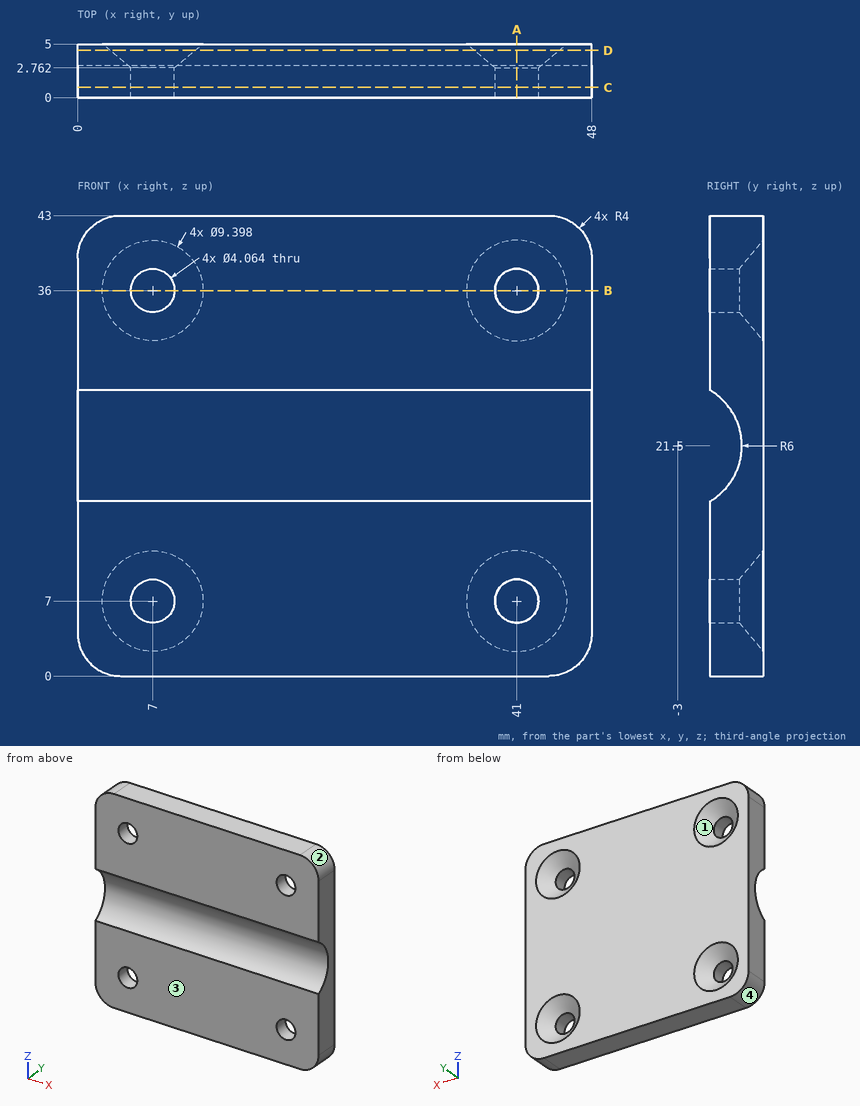
Verification items for this drawing (mm, ordinates from the low corner). Coordinates: 2 decimals unless noted, no trailing zeros. Loops run counter-clockwise (first coordinate to the right, second up) from the corner with the lowest first, then second, coordinate; pieces in that order, holes last.
Item 1: Sectioned sample at C-C, the plane y = 0.95. Record the boundary of the cut face in (x, z), then the cut area to 3 significant figures.
Item 2: Go/stop test with a flat-tipped pin: pin 1 Ø4.5 at (x, z) = (7, 7) entering from -Y. Record where the tip stops, or that it passes through.
Item 3: Release check for a two-part mould opening along Z. For the marked faces 1, 2, 3 and 4 record: released by +Z, released by -Z, zero draft, split by the parting line, or undercut.
Item 4: Thickness scan on line 1 (X direction, y = 1.5, z = 7); line 2 (X direction, y = 3.45, z = 35); line 3 (Z direction, x = 41, y = 1.9). Record the ranges inside material, lowest first.
Item 5: Sectioned sample at B-B, the plane z = 36. Record the boundary of the cut face in (x, y), then the cut area to 3 significant figures.
Item 6: Sectioned sample at A-A, the plane x = 41. Record the boundary of the cut face in (y, z).
Item 7: Sectioned sample at D-D, the plane y = 4.4. Record the boundary of the cut face in (x, z).
Check result:
1. outline: (0, 4) arc R4 ccw to (4, 0) - (44, 0) arc R4 ccw to (48, 4) - (48, 16.98) - (0, 16.98) - close; (0, 26.02) - (48, 26.02) - (48, 39) arc R4 ccw to (44, 43) - (4, 43) arc R4 ccw to (0, 39) - close; hole circle Ø4.06 at (7, 7); hole circle Ø4.06 at (7, 36); hole circle Ø4.06 at (41, 7); hole circle Ø4.06 at (41, 36)
1. area: 1,560 mm2
2. pin 1: stops at y = 0
3. face 1: undercut
3. face 2: released by +Z
3. face 3: zero draft
3. face 4: released by -Z
4. line 1: x = 0 to 4.97, 9.03 to 38.97, 43.03 to 48
4. line 2: x = 0 to 4.33, 9.67 to 38.33, 43.67 to 48
4. line 3: z = 0 to 4.97, 9.03 to 18.04, 24.96 to 33.97, 38.03 to 43
5. outline: (0, 0) - (4.97, 0) - (4.97, 2.76) - (2.3, 5) - (0, 5) - close; (9.03, 0) - (38.97, 0) - (38.97, 2.76) - (36.3, 5) - (11.7, 5) - (9.03, 2.76) - close; (43.03, 0) - (48, 0) - (48, 5) - (45.7, 5) - (43.03, 2.76) - close
5. area: 187 mm2
6. outline: (0, 0) - (5, 0) - (5, 2.3) - (2.76, 4.97) - (0, 4.97) - close; (0, 9.03) - (2.76, 9.03) - (5, 11.7) - (5, 31.3) - (2.76, 33.97) - (0, 33.97) - (0, 26.7) arc R6 cw to (0, 16.3) - close; (0, 38.03) - (2.76, 38.03) - (5, 40.7) - (5, 43) - (0, 43) - close
7. outline: (0, 4) arc R4 ccw to (4, 0) - (44, 0) arc R4 ccw to (48, 4) - (48, 39) arc R4 ccw to (44, 43) - (4, 43) arc R4 ccw to (0, 39) - close; hole circle Ø7.97 at (7, 7); hole circle Ø7.97 at (7, 36); hole circle Ø7.97 at (41, 7); hole circle Ø7.97 at (41, 36)
